```python
from build123d import *

# Parameters (mm, degrees)
SKETCH1_W                       = 56
SKETCH1_H                       = 56
BASE_FLANGE1_DEPTH              = 28
SKETCH6_R                       = 19
SKETCH6_R_2                     = 2.5
CUT_EXTRUDE1_DEPTH              = 49.497422612
FILLET1_R                       = 5
M4X0_7_TAPPED_HOLE1_D           = 3.3
M4X0_7_TAPPED_HOLE1_DEPTH       = 12.1
M4X0_7_TAPPED_HOLE1_CSINK_D     = 4.05
M4X0_7_TAPPED_HOLE1_CSINK_ANGLE = 90
M4X0_7_TAPPED_HOLE1_TIP         = 0.991420021


# Sheet-metal steps are written as plain solids
with BuildPart() as part:
    # Sketch1 → Base-Flange1 (new body)
    with BuildSketch(Plane.XY):
        Rectangle(SKETCH1_W, SKETCH1_H)
    extrude(amount=-BASE_FLANGE1_DEPTH)

    # Sketch6 → Cut-Extrude1 (cut, through all)
    with BuildSketch(Plane.XY):
        Circle(SKETCH6_R)
        with Locations((-23.5, 23.5)):
            Circle(SKETCH6_R_2)
        with Locations((23.5, 23.5)):
            Circle(SKETCH6_R_2)
        with Locations((23.5, -23.5)):
            Circle(SKETCH6_R_2)
        with Locations((-23.5, -23.5)):
            Circle(SKETCH6_R_2)
    extrude(amount=-CUT_EXTRUDE1_DEPTH, mode=Mode.SUBTRACT)

    # Fillet1
    fillet1_edges = [part.edges().sort_by_distance(p)[0] for p in [
        (28, -28, -14),
        (-28, -28, -14),
        (-28, 28, -14),
        (28, 28, -14),
    ]]
    fillet(fillet1_edges, radius=FILLET1_R)

    # M4x0.7 Tapped Hole1
    with Locations(Plane.XY):
        with Locations((0, 22), (-22, 0), (0, -22), (22, 0)):
            CounterSinkHole(M4X0_7_TAPPED_HOLE1_D / 2, M4X0_7_TAPPED_HOLE1_CSINK_D / 2, depth=M4X0_7_TAPPED_HOLE1_DEPTH, counter_sink_angle=M4X0_7_TAPPED_HOLE1_CSINK_ANGLE)
            with Locations((0, 0, -(M4X0_7_TAPPED_HOLE1_DEPTH + M4X0_7_TAPPED_HOLE1_TIP / 2))):  # 118° drill point
                Cone(0, M4X0_7_TAPPED_HOLE1_D / 2, M4X0_7_TAPPED_HOLE1_TIP, mode=Mode.SUBTRACT)


solid = part.part
```
Design review of the part built by this model. Coordinates are the model's own, in mm. A direction names the side the tool comes from. Round coordinates to 2 decimals unless told otherwise and drop trailing zeros. Write each loop counter-clockwise with the first axis right and the second up, starting at its lowest first coordinate (ties: lowest second). Pieces come first, ordered by that corner, then holes. Notation, with made-up numbers: (14.25, 9) -> (38.25, 9) arc R18 ccw to (38.25, 34) -> close; hole circle Ø9 at (1, 77.5). An arc over 180 degrees is marked (long way). Write item = value, one per line. Start each with the question number.
1) Take a section at D-D, the plane y = 15. State the section outline as (x, z) points, plus the area to 3 significant figures.
2) Take a section at B-B, the plane z = -8. Count the separate pieces of the cut face and the enclosed holes in it, plus the area to 3 significant figures.
3) Tool access review of faces 1 (the face through (0.215, -20.364, -6.32)), 2 (the face through (-25.34, -21.81, -13.8)): name each direction out of +Z, -Z, +X, -X, +Y, -Y from which nothing blocks a thin tool from reaching the whole face with its end or side.
4) Take a section at A-A, the plane z = -14.25. State the section outline as (x, y) points, plus the area to 3 significant figures.
5) Take a section at C-C, the plane x = 5.5. State the section outline as (y, z) points.
6) Wall thickness on probe 1 along Y at (x, z) = (0, -7); probe 2 along Y at (x, z) = (0, -18); probe 3 along X at (y, z) = (-0.5, -10): over which ranges is each line inside the solid? List them lowest first. Write a range as from..to.
7) Mouldability with a two-part tool opening along X and no side actions: class faces 3 (the face through (0, -28, -14)), 4 (the face through (-28, 0, -14)), 5 (the face through (-20.35, 0.07, -6.32)) as +X half, -X half, draft (parallel to the pull), parting line (faces both ways), or undercut.
Results list:
q1.outline = (-28, -28) -> (-11.66, -28) -> (-11.66, 0) -> (-28, 0) -> close; (11.66, -28) -> (28, -28) -> (28, 0) -> (11.66, 0) -> close
q1.area = 915 mm²
q2.separate_pieces = 1
q2.enclosed_holes = 9
q2.area = 1,870 mm²
q3.face_1 = +Z
q3.face_2 = +Z, -Z
q4.outline = (-28, -23) arc R5 ccw to (-23, -28) -> (23, -28) arc R5 ccw to (28, -23) -> (28, 23) arc R5 ccw to (23, 28) -> (-23, 28) arc R5 ccw to (-28, 23) -> close; hole circle Ø5 at (-23.5, -23.5); hole circle Ø5 at (-23.5, 23.5); hole circle Ø38 at (0, 0); hole circle Ø5 at (23.5, -23.5); hole circle Ø5 at (23.5, 23.5)
q4.area = 1,900 mm²
q5.outline = (-28, -28) -> (-18.19, -28) -> (-18.19, 0) -> (-28, 0) -> close; (18.19, -28) -> (28, -28) -> (28, 0) -> (18.19, 0) -> close
q6.probe_1 = -28..-23.65, -20.35..-19, 19..20.35, 23.65..28
q6.probe_2 = -28..-19, 19..28
q6.probe_3 = -28..-23.57, -20.43..-18.99, 18.99..20.43, 23.57..28
q7.face_3 = draft
q7.face_4 = -X half
q7.face_5 = undercut
